Here's how the part is built. I have some questions about the finished solid (model axes, mm). A direction names the side the tool comes from. Give positions to 0.01 mm unless a question says otherwise; leave off trailing zeros. Loops run counter-clockwise (first coordinate to the right, second up) from the corner with the lowest first, then second, coordinate; pieces in that order, holes last.
Q1. We'd pull the mould along Y, two halves only. Please class faces 1 (the face through (317.68, -54.62, 390.47)), 2 (the face through (355.6, 74, 231)), 3 (the face through (343.078, 142.429, 315.707)): +Y half, -Y half, draft (parallel to the pull), parting line (faces both ways), or undercut.
Q2. I need wall thicknesses on line 1 (Y direction, x = 337, z = 341); line 2 (Z direction, x = 338, y = -37); line 3 (Z direction, x = 333, y = 41). Which ranges of each line are inside material? Lowest first, please.
Q3. For faces 4 (the face through (304.8, -45, 222)), 5 (the face through (330.2, 74, 231)), which set-ups out of +Z, -Z, +X, -X, +Y, -Y let a thin tool reach every point of the face, with its end or its side?
Q4. If we section it at B-B (z = 304.8): Please give me the cut outline in (x, y).
Q5. Will these pins go through, and if not, where does the flat tip stop? P1, Ø1.5, axis at x = 310.5, z = 273.5, coming from the -Y side; P2, Ø4, axis at x = 340, z = 339.5, coming from the +Y side; P3, Ø23, axis at y = -120.22, z = 236.32, coming from the +X side; P4, Ø1, axis at x = 326.5, y = -22, coming from the -Z side.
Q6. If we section it at D-D (z = 228.5): Please give me the cut outline in (x, y), plus the area to 3 significant figures.
Q7. If we section it at A-A (y = 0): Please give me the cut outline in (x, z).
Q8. If we section it at C-C (x = 349.5): Give the number of separate pieces and of enclosed holes in the cut face, plus the area to 3 significant figures.
from build123d import *

# Parameters (mm, degrees)
F0_R      = 101.6
F0_R_2    = 93.4212
F3_DEPTH  = 25.4
F4_R      = 171.45
F4_R_2    = 93.4212
F5_DEPTH  = 25.4
F6_SIZE   = 5.08
F7_R      = 12.7
F8_DEPTH  = 457.1692501
F10_R     = 101.6
F10_R_2   = 93.4212
F11_DEPTH = 25.4


with BuildPart() as f2:
    # F2: sweep along a path in F1
    with BuildLine(Plane.XZ) as f2_path:
        ThreePointArc((0, 0), (89.2738530943, 215.5261469057), (304.8, 304.8))
    # F0 (on Top) → F2 (sweep)
    with BuildSketch(Plane.XY):
        Circle(F0_R)
        Circle(F0_R_2, mode=Mode.SUBTRACT)
    sweep(path=f2_path.line)

    # F3 (add): a face of the model
    f3_faces = [f2.faces().sort_by_distance(p)[0] for p in [
        (304.8, 0, 403.5263180413),
    ]]
    extrude(f3_faces, amount=F3_DEPTH)

    # F6
    f6_edges = [f2.edges().sort_by_distance(p)[0] for p in [
        (-101.6, 0, 0),
    ]]
    chamfer(f6_edges, length=F6_SIZE)


with BuildPart() as f5:
    # F4 (on face) → F5 (new body)
    with BuildSketch(Plane.YZ.offset(330.2)):
        with Locations((0, 304.8)):
            Circle(F4_R)
        with Locations((0, 304.8)):
            Circle(F4_R_2, mode=Mode.SUBTRACT)
    extrude(amount=F5_DEPTH)


with BuildPart() as f8_tool:
    # F7 (on face) → F8 (new body, through all)
    with BuildSketch(Plane.YZ.offset(355.6)):
        with Locations((-88.7286911595, 410.9601527047)):
            Circle(F7_R)
        with Locations((0, 443.1573585219)):
            Circle(F7_R)
        with Locations((90.5679274826, 409.3954548185)):
            Circle(F7_R)
        with Locations((136.5689763149, 326.9737088793)):
            Circle(F7_R)
        with Locations((119.0079640377, 234.2318545463)):
            Circle(F7_R)
        with Locations((46.0581534638, 174.3338926898)):
            Circle(F7_R)
        with Locations((-48.328086115, 175.1575889239)):
            Circle(F7_R)
        with Locations((-120.2214225043, 236.3195777744)):
            Circle(F7_R)
        with Locations((-136.1611916187, 329.3537889975)):
            Circle(F7_R)
    extrude(amount=-F8_DEPTH)


with BuildPart() as f2_1:
    add(f2.part)

    # F8: cut by f8_tool
    add(f8_tool.part, mode=Mode.SUBTRACT)


with BuildPart() as f5_1:
    add(f5.part)

    # F8: cut by f8_tool
    add(f8_tool.part, mode=Mode.SUBTRACT)

    # F10 (on face) → F11 (join)
    with BuildSketch(Plane(origin=(330.2, 0, 0), x_dir=(0, -1, 0), z_dir=(-1, 0, 0))):
        with Locations((0, 304.8)):
            Circle(F10_R)
        with Locations((0, 304.8)):
            Circle(F10_R_2, mode=Mode.SUBTRACT)
    extrude(amount=F11_DEPTH)


solid = f5_1.part
Check sheet entries:
1. face 1: parting line
1. face 2: draft
1. face 3: undercut
2. line 1: y = -167.58 to -141.23, -131.1 to -86.12, 86.12 to 167.58
2. line 2: z = 137.39 to 169.42, 180.9 to 219.02, 390.58 to 472.21
2. line 3: z = 138.32 to 162.68, 185.98 to 220.86, 388.74 to 471.28
3. face 4: +Z, -Z, -X, +Y, -Y
3. face 5: -X
4. outline: (304.8, -101.6) - (330.2, -101.6) - (330.2, -171.45) - (355.6, -171.45) - (355.6, -93.42) - (304.8, -93.42) - close; (304.8, 93.42) - (355.6, 93.42) - (355.6, 171.45) - (330.2, 171.45) - (330.2, 101.6) - (304.8, 101.6) - close
5. P1: stops at y = -96.9
5. P2: stops at y = 168.3
5. P3: passes through
5. P4: stops at z = 205.5
6. outline: (304.8, -67.09) - (330.2, -67.09) - (330.2, -110.21) - (355.6, -110.21) - (355.6, -53.91) - (304.8, -53.91) - close; (304.8, 53.91) - (355.6, 53.91) - (355.6, 107.68) - (330.2, 107.68) - (330.2, 67.09) - (304.8, 67.09) - close; (330.2, -153.54) - (355.6, -153.54) - (355.6, -130.23) - (330.2, -130.23) - close; (330.2, 130.34) - (355.6, 130.34) - (355.6, 153.54) - (330.2, 153.54) - close
6. area: 4,650 mm2
7. outline: (304.8, 203.2) - (330.2, 203.2) - (330.2, 133.35) - (355.6, 133.35) - (355.6, 211.38) - (304.8, 211.38) - close; (304.8, 398.22) - (355.6, 398.22) - (355.6, 430.46) - (330.2, 430.46) - (330.2, 406.4) - (304.8, 406.4) - close; (330.2, 455.86) - (355.6, 455.86) - (355.6, 476.25) - (330.2, 476.25) - close
8. separate pieces: 1
8. enclosed holes: 10
8. area: 60,400 mm2
